Read the model definition and answer for the solid it produces. Units are mm, in the model's axes. A direction names the side the tool comes from. Coordinates: 2 decimals unless noted, no trailing zeros. Write each loop counter-clockwise with the first axis right and the second up, starting at its lowest first coordinate (ties: lowest second). Pieces come first, ordered by that corner, then holes. Notation, with made-up numbers: (-13, 77) -> (8, 77) arc R15 cw to (8, 99) -> close; hole circle Ø4 at (82, -17.5). An arc over 180 degrees is marked (long way). Return JSON: item names as keys, results as strings.
from build123d import *

# Parameters (mm, degrees)
BOSS_EXTRUDE1_DEPTH         = 12.7
BOSS_EXTRUDE1_DEPTH_BACK    = 12.7
F_1_4_0_25_DIAMETER_HOLE1_D = 6.35
SKETCH6_W                   = 152.4
SKETCH6_H                   = 6.35
BOSS_EXTRUDE2_DEPTH         = 75
BOSS_EXTRUDE2_DEPTH_BACK    = 75
CHAMFER1_SIZE               = 7.5


with BuildPart() as part:
    # Sketch-Profile → Boss-Extrude1 (new body, two sides)
    with BuildSketch(Plane(origin=(0, 0, 0), x_dir=(0, 0, -1), z_dir=(1, 0, 0))) as boss_extrude1_sk:
        Polygon((-76.2, 6.35), (-76.2, 0), (76.2, 0), (76.2, 6.35), (19.05, 6.35), (19.05, 50.8), (-19.05, 50.8), (-19.05, 6.35), align=None)
    extrude(amount=BOSS_EXTRUDE1_DEPTH)
    extrude(boss_extrude1_sk.sketch, amount=-BOSS_EXTRUDE1_DEPTH_BACK)

    # 1_4 _0.25_ Diameter Hole1 (through all)
    with Locations(Plane.XY.offset(19.05)):
        with Locations((0, 27.5181)):
            Hole(F_1_4_0_25_DIAMETER_HOLE1_D / 2)

    # Sketch6 → Boss-Extrude2 (add, two sides)
    with BuildSketch(Plane(origin=(0, 0, 0), x_dir=(0, 0, -1), z_dir=(1, 0, 0))) as boss_extrude2_sk:
        with Locations((0, 3.175)):
            Rectangle(SKETCH6_W, SKETCH6_H)
    extrude(amount=BOSS_EXTRUDE2_DEPTH)
    extrude(boss_extrude2_sk.sketch, amount=-BOSS_EXTRUDE2_DEPTH_BACK)

    # Chamfer1
    chamfer1_edges = [part.edges().sort_by_distance(p)[0] for p in [
        (0, 6.35, 19.05),
        (0, 6.35, -19.05),
        (12.7, 6.35, 0),
        (-12.7, 6.35, 0),
    ]]
    chamfer(chamfer1_edges, length=CHAMFER1_SIZE)


solid = part.part
1. Consider L1, parallel to Y at x = 0, z = 6; L2, parallel to Y at x = -1, z = 61.5; L3, parallel to X at y = 46.5, z = -11. Determine where each line is inside the solid, lowest interval first.
Taken from the geometry:
{"L1": "y = 0 to 24.34, 30.69 to 50.8", "L2": "y = 0 to 6.35", "L3": "x = -12.7 to 12.7"}
2. For a pull along Y with two mould halves and no side action, classify faces 1 (the face through (-1.465, 24.701, -0.267)), 2 (the face through (-16.4, 10.15, 0.37)), 3 (the face through (1, 3, -76.2)) as +Y half, -Y half, draft (parallel to the pull), parting line (faces both ways), or undercut.
Taken from the geometry:
{"face 1": "undercut", "face 2": "+Y half", "face 3": "draft"}
3. The part is cut by section B-B (x = 17). Determine the outline of the cut face in (y, z).
Taken from the geometry:
{"outline": "(0, -76.2) -> (6.35, -76.2) -> (6.35, -26.55) -> (9.55, -23.35) -> (9.55, 23.35) -> (6.35, 26.55) -> (6.35, 76.2) -> (0, 76.2) -> close"}
4. The part is cut by section C-C (z = 3.5). Determine the outline of the cut face in (x, y) (3 decimals), then the cut area to 3 significant figures.
Taken from the geometry:
{"outline": "(-75, 0) -> (75, 0) -> (75, 6.35) -> (20.2, 6.35) -> (12.7, 13.85) -> (12.7, 50.8) -> (-12.7, 50.8) -> (-12.7, 13.85) -> (-20.2, 6.35) -> (-75, 6.35) -> close; hole circle Ø6.35 at (0, 27.518)", "area": "2,110 mm2"}
5. Flat-ended cylindrical pins translate along their axes: pin 1 Ø7.5 at (x, y) = (2, 33.5) entering from +Z; pin 2 Ø12 at (x, z) = (42, -51) entering from +Y; pin 3 Ø5 at (x, y) = (0, 27.52) entering from +Z; pin 4 Ø18.5 at (y, z) = (40.5, -1.5) entering from -X. Find the tip coordinate at first contact, or state that the pin passes through.
Taken from the geometry:
{"pin 1": "stops at z = 19.05", "pin 2": "stops at y = 6.35", "pin 3": "passes through", "pin 4": "stops at x = -12.7"}
6. A tool of negligible diameter and unlimited length cuts with its end or side. For faces 4 (the face through (-12.7, 33, 0)), 5 (the face through (0, 32, -19.05)), 6 (the face through (0, 33, 19.05)), 7 (the face through (12.7, 33, 0)), from which of +Z, -Z, +X, -X, +Y, -Y can it reach the whole face along a straight path? Write none if from no direction.
Taken from the geometry:
{"face 4": "+Z, -Z, -X, +Y", "face 5": "-Z, +X, -X, +Y", "face 6": "+Z, +X, -X, +Y", "face 7": "+Z, -Z, +X, +Y"}
7. The part is cut by section A-A (x = 0). Determine the outline of the cut face in (y, z), then the cut area to 3 significant figures.
Taken from the geometry:
{"outline": "(0, -76.2) -> (6.35, -76.2) -> (6.35, -26.55) -> (13.85, -19.05) -> (24.34, -19.05) -> (24.34, 19.05) -> (13.85, 19.05) -> (6.35, 26.55) -> (6.35, 76.2) -> (0, 76.2) -> close; (30.69, -19.05) -> (50.8, -19.05) -> (50.8, 19.05) -> (30.69, 19.05) -> close", "area": "2,480 mm2"}
8. The part is cut by section D-D (y = 34). Determine the outline of the cut face in (x, z).
Taken from the geometry:
{"outline": "(-12.7, -19.05) -> (12.7, -19.05) -> (12.7, 19.05) -> (-12.7, 19.05) -> close"}
